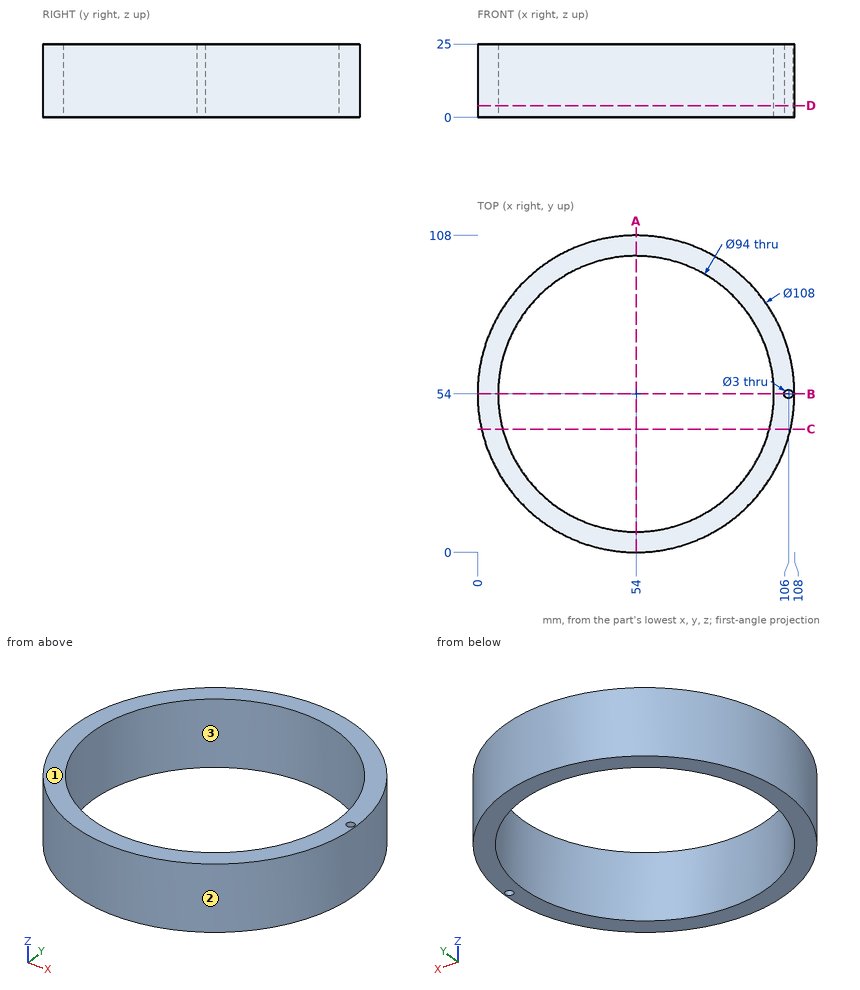
Verification items for this drawing (mm, ordinates from the low corner). Coordinates: 2 decimals unless noted, no trailing zeros. Order: outer loops, then holes, each group sorted by start corner. A loop starts at its lowest first (then second) coordinate and runs counter-clockwise, first axis right, second up. Notation, with made-up numbers: M -3.75,0 L 27.25,0 A29 cw 27.25,27 Z; hole C 72.25,-24.75 d8. An arc over 180 degrees is marked long. Write each question's results on one line, items separated by ' | '.
1) Section check A-A on x = 54. Record the cut outline in (y, z).
Solved:
outline: M 0,0 L 7,0 L 7,25 L 0,25 Z; M 101,0 L 108,0 L 108,25 L 101,25 Z
2) Release check for a two-part mould opening along Y. For the marked faces 1, 2 and 3 record: pulls with the +Y half, pulls with the -Y half, needs draft (parallel to the pull), parting line crosses it, or undercut.
Solved:
face 1: needs draft | face 2: parting line crosses it | face 3: undercut
3) Section check C-C on y = 42. Record the cut outline in (x, z), plus the area to 3 significant figures.
Solved:
outline: M 1.35,0 L 8.56,0 L 8.56,25 L 1.35,25 Z; M 99.44,0 L 106.65,0 L 106.65,25 L 99.44,25 Z | area: 360 mm²
4) Gauge pin test, flat ends, axial feed: pin 1 Ø10 at (x, z) = (56, 7.5) entering from -Y; pin 2 Ø3 at (y, z) = (45, 6) entering from -X; pin 3 Ø8 at (y, z) = (64, 16) entering from -X. Record the tip position at first contact, or that the pin passes through.
Solved:
pin 1: stops at y = 0 | pin 2: stops at x = 0.52 | pin 3: stops at x = 0.33
5) Scan lines: line 1 along Y through (x, z) = (54, 8); line 2 along Y through (x, z) = (72.5, 2); line 3 along X through (y, z) = (40, 22.75). Record each from-to range of solid material in increasing order. Write a range as [from, to].
Solved:
line 1: y = [0, 7], [101, 108] | line 2: y = [3.27, 10.79], [97.21, 104.73] | line 3: x = [1.85, 9.13], [98.87, 106.15]
6) Section check B-B on y = 54. Record the cut outline in (x, z).
Solved:
outline: M 0,0 L 7,0 L 7,25 L 0,25 Z; M 101,0 L 104.5,0 L 104.5,25 L 101,25 Z; M 107.5,0 L 108,0 L 108,25 L 107.5,25 Z
7) Section check D-D on z = 4. Record the cut outline in (x, y), plus the area to 3 significant figures.
Solved:
outline: C 54,54 d108; hole C 54,54 d94; hole C 106,54 d3 | area: 2,210 mm²
